Read the model definition and answer for the solid it produces. Units are mm, in the model's axes. Face numbers are marked on the shaded views. A direction names the side the tool comes from. Give positions to 0.01 mm unless a question says otherwise; leave off trailing zeros. Order: outer loops, then holes, each group sorted by start corner. A loop starts at its lowest first (then second) coordinate and runs counter-clockwise, first axis right, second up. Notation, with made-up numbers: (54.25, 88.25) - (86.25, 88.25) arc R25 ccw to (86.25, 103.25) - close; hole circle Ø4 at (-17.75, 21). An arc over 180 degrees is marked (long way). Write each question's results on one line, items separated by ' | '.
from build123d import *

# Parameters (mm, degrees)
BOSS_EXTRUDE3_DEPTH = 2
SKETCH1_6_W         = 100
SKETCH1_6_H         = 50
BOSS_EXTRUDE4_DEPTH = 5
SKETCH2_W           = 120
SKETCH2_H           = 65
SKETCH2_R           = 1.45
SKETCH2_R_2         = 1.6
BOSS_EXTRUDE5_DEPTH = 30
SKETCH2_2_W         = 120
SKETCH2_2_H         = 65
SKETCH2_2_R         = 1.45
SKETCH2_2_R_2       = 1.6
BOSS_EXTRUDE6_DEPTH = 3
CUT_EXTRUDE1_REACH  = 77.367
SKETCH7_W           = 43
SKETCH7_H           = 32
FILLET1_R           = 10


with BuildPart() as part:
    # Sketch1 → Boss-Extrude3 (new body)
    with BuildSketch(Plane(origin=(0, 0, 0), x_dir=(1, 0, 0), z_dir=(0, 1, 0))):
        Polygon((23, -14.25), (23, -17.5), (-23, -17.5), (-23, -14.25), (-38.5, -14.25), (-38.5, 14.25), (-23, 14.25), (-23, 17.5), (23, 17.5), (23, 14.25), (38.5, 14.25), (38.5, -14.25), align=None)
    extrude(amount=BOSS_EXTRUDE3_DEPTH)

    # Sketch1<6> → Boss-Extrude4 (add)
    with BuildSketch(Plane(origin=(0, 0, 0), x_dir=(1, 0, 0), z_dir=(0, 1, 0))):
        Rectangle(SKETCH1_6_W, SKETCH1_6_H)
        Polygon((23, -14.25), (23, -17.5), (-23, -17.5), (-23, -14.25), (-38.5, -14.25), (-38.5, 14.25), (-23, 14.25), (-23, 17.5), (23, 17.5), (23, 14.25), (38.5, 14.25), (38.5, -14.25), align=None, mode=Mode.SUBTRACT)
    extrude(amount=BOSS_EXTRUDE4_DEPTH)

    # Sketch2 → Boss-Extrude5 (add)
    with BuildSketch(Plane.XZ):
        Rectangle(SKETCH2_W, SKETCH2_H)
        with Locations(Location((-55, 28.75, 0), (0, 0, 270))):
            Circle(SKETCH2_R, mode=Mode.SUBTRACT)
        with Locations(Location((55, 28.75, 0), (0, 0, 90))):
            Circle(SKETCH2_R, mode=Mode.SUBTRACT)
        with Locations(Location((55, -28.75, 0), (0, 0, 270))):
            Circle(SKETCH2_R, mode=Mode.SUBTRACT)
        with Locations(Location((-55, -28.75, 0), (0, 0, 90))):
            Circle(SKETCH2_R, mode=Mode.SUBTRACT)
        with Locations(Location((50, 28.75, 0), (0, 0, 270))):
            Circle(SKETCH2_R_2, mode=Mode.SUBTRACT)
        with Locations(Location((50, -28.75, 0), (0, 0, 90))):
            Circle(SKETCH2_R_2, mode=Mode.SUBTRACT)
    extrude(amount=BOSS_EXTRUDE5_DEPTH)

    # Sketch2<2> → Boss-Extrude6 (add)
    with BuildSketch(Plane.XZ):
        Rectangle(SKETCH2_2_W, SKETCH2_2_H)
        with Locations(Location((-55, 28.75, 0), (0, 0, 270))):
            Circle(SKETCH2_2_R, mode=Mode.SUBTRACT)
        with Locations(Location((55, 28.75, 0), (0, 0, 90))):
            Circle(SKETCH2_2_R, mode=Mode.SUBTRACT)
        with Locations(Location((55, -28.75, 0), (0, 0, 270))):
            Circle(SKETCH2_2_R, mode=Mode.SUBTRACT)
        with Locations(Location((-55, -28.75, 0), (0, 0, 90))):
            Circle(SKETCH2_2_R, mode=Mode.SUBTRACT)
        with Locations(Location((50, 28.75, 0), (0, 0, 270))):
            Circle(SKETCH2_2_R_2, mode=Mode.SUBTRACT)
        with Locations(Location((50, -28.75, 0), (0, 0, 90))):
            Circle(SKETCH2_2_R_2, mode=Mode.SUBTRACT)
    extrude(amount=BOSS_EXTRUDE6_DEPTH)

    # Sketch7 → Cut-Extrude1 (cut, up to next)
    with BuildSketch(Plane(origin=(0, 2, 0), x_dir=(1, 0, 0), z_dir=(0, 1, 0)), mode=Mode.PRIVATE) as cut_extrude1_sk1:
        Rectangle(SKETCH7_W, SKETCH7_H)
    cut_extrude1_tool1 = extrude(cut_extrude1_sk1.sketch, amount=-CUT_EXTRUDE1_REACH, mode=Mode.PRIVATE) & part.part
    add(cut_extrude1_tool1.solids().sort_by_distance((0, 2, 0))[0], mode=Mode.SUBTRACT)

    # Fillet1
    # the kernel refuses this fillet: 10 mm, written as the material it takes off along each edge
    with BuildSketch(Plane(origin=(-21.5, 2, 16), x_dir=(0, -1, 0), z_dir=(0, 0, -1))) as fillet1_piece_1_section:
        with BuildLine():
            CenterArc((FILLET1_R, FILLET1_R), FILLET1_R, 180, 90)
            Line((0, FILLET1_R), (0, 0))
            Line((0, 0), (FILLET1_R, 0))
        make_face()
    fillet1_piece_1 = extrude(amount=32, mode=Mode.PRIVATE)
    fillet1_piece_1 = split(fillet1_piece_1, bisect_by=Plane(origin=(-23, -2.387167078, 15.125), z_dir=(1, 0, 0)), keep=Keep.TOP, mode=Mode.PRIVATE)
    add(fillet1_piece_1, mode=Mode.SUBTRACT)
    with BuildSketch(Plane(origin=(-21.5, 2, 41), x_dir=(0, -1, 0), z_dir=(0, 0, -1))) as fillet1_piece_2_section:
        with BuildLine():
            CenterArc((FILLET1_R, FILLET1_R), FILLET1_R, 180, 90)
            Line((0, FILLET1_R), (0, 0))
            Line((0, 0), (FILLET1_R, 0))
        make_face()
    fillet1_piece_2 = extrude(amount=82, mode=Mode.PRIVATE)
    fillet1_piece_2 = split(fillet1_piece_2, bisect_by=Plane(origin=(-23.780995079, -0.852225246, -14.25), z_dir=(0, 0, 1)), keep=Keep.TOP, mode=Mode.PRIVATE)
    fillet1_piece_2 = split(fillet1_piece_2, bisect_by=Plane(origin=(-23.780995079, -0.852225246, 14.25), z_dir=(0, 0, -1)), keep=Keep.TOP, mode=Mode.PRIVATE)
    add(fillet1_piece_2, mode=Mode.SUBTRACT)
    with BuildSketch(Plane(origin=(21.5, 2, -16), x_dir=(0, -1, 0), z_dir=(0, 0, 1))) as fillet1_piece_3_section:
        with BuildLine():
            CenterArc((FILLET1_R, FILLET1_R), FILLET1_R, 180, 90)
            Line((0, FILLET1_R), (0, 0))
            Line((0, 0), (FILLET1_R, 0))
        make_face()
    fillet1_piece_3 = extrude(amount=32, mode=Mode.PRIVATE)
    fillet1_piece_3 = split(fillet1_piece_3, bisect_by=Plane(origin=(23, -2.387167078, -15.125), z_dir=(-1, 0, 0)), keep=Keep.TOP, mode=Mode.PRIVATE)
    add(fillet1_piece_3, mode=Mode.SUBTRACT)
    with BuildSketch(Plane(origin=(21.5, 2, -41), x_dir=(0, -1, 0), z_dir=(0, 0, 1))) as fillet1_piece_4_section:
        with BuildLine():
            CenterArc((FILLET1_R, FILLET1_R), FILLET1_R, 180, 90)
            Line((0, FILLET1_R), (0, 0))
            Line((0, 0), (FILLET1_R, 0))
        make_face()
    fillet1_piece_4 = extrude(amount=82, mode=Mode.PRIVATE)
    fillet1_piece_4 = split(fillet1_piece_4, bisect_by=Plane(origin=(23.780995079, -0.852225246, 14.25), z_dir=(0, 0, -1)), keep=Keep.TOP, mode=Mode.PRIVATE)
    fillet1_piece_4 = split(fillet1_piece_4, bisect_by=Plane(origin=(23.780995079, -0.852225246, -14.25), z_dir=(0, 0, 1)), keep=Keep.TOP, mode=Mode.PRIVATE)
    add(fillet1_piece_4, mode=Mode.SUBTRACT)


solid = part.part
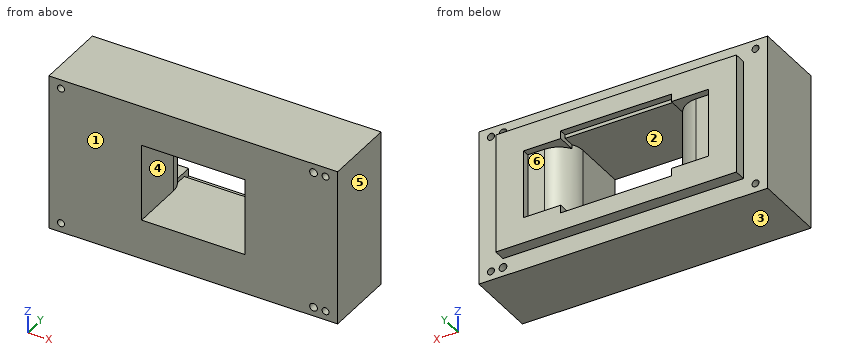
(1) The mould has two halves that part along Z. Classify the marked faces 1, 2 and 3: pulls with the +Z half, pulls with the -Z half, needs draft (parallel to the pull), parting line crosses it, or undercut.
Conclusion:
face 1: needs draft | face 2: undercut | face 3: pulls with the -Z half
(2) Section B-B (y = -15) is taken. Give the vertices of the cut face in (x, z), plus the area to 3 significant figures.
Conclusion:
outline: (-60, -32.5) - (60, -32.5) - (60, 32.5) - (-60, 32.5) - close; hole circle Ø2.9 at (-55, -28.75); hole circle Ø2.9 at (-55, 28.75); hole (-21.5, -16) - (21.5, -16) - (21.5, 16) - (-21.5, 16) - close; hole circle Ø3.2 at (50, -28.75); hole circle Ø3.2 at (50, 28.75); hole circle Ø2.9 at (55, -28.75); hole circle Ø2.9 at (55, 28.75) | area: 6,380 mm^2
(3) Section C-C (x = -55) is taken. Give the vertices of the cut face in (y, z).
Conclusion:
outline: (-30, -32.5) - (0, -32.5) - (0, -30.2) - (-30, -30.2) - close; (-30, -27.3) - (0, -27.3) - (0, 27.3) - (-30, 27.3) - close; (-30, 30.2) - (0, 30.2) - (0, 32.5) - (-30, 32.5) - close
(4) Each of these flat-tipped pins is pushed along its axis until it touches: pin 1 (1.5 mm diameter, centred on y = 3.5, z = 4.5, fed in from -X); pin 2 (4 mm diameter, centred on x = 50, z = -28.75, fed in from +Y); pin 3 (1.5 mm diameter, centred on y = 3, z = -3.5, fed in from +X); pin 4 (5 mm diameter, centred on x = -18, z = 4, fed in from -Y) (1 decimal). Where does it stop, or does it pass through?
Conclusion:
pin 1: x = -50 | pin 2: y = 0 | pin 3: x = 50 | pin 4: through
(5) For the marked faces 4, 5 and 6, determine the directions among +Z, -Z, +X, -X, +Y, -Y from which every point of the face is accessible in a straight line to the end or side of a thin tool.
Conclusion:
face 4: +Y, -Y | face 5: +Z, -Z, +X, +Y, -Y | face 6: +Y
(6) Section D-D (z = -28.75) is taken. Give the vertices of the cut face in (x, y), plus the area to 3 significant figures.
Conclusion:
outline: (-60, -30) - (-56.45, -30) - (-56.45, 0) - (-60, 0) - close; (-53.55, -30) - (48.4, -30) - (48.4, 0) - (-53.55, 0) - close; (51.6, -30) - (53.55, -30) - (53.55, 0) - (51.6, 0) - close; (56.45, -30) - (60, -30) - (60, 0) - (56.45, 0) - close | area: 3,330 mm^2
(7) Section A-A (z = 1) is taken. Give the vertices of the cut face in (x, y).
Conclusion:
outline: (-60, -30) - (-21.5, -30) - (-21.5, -8) arc R10 ccw to (-31.5, 2) - (-38.5, 2) - (-38.5, 5) - (-50, 5) - (-50, 0) - (-60, 0) - close; (21.5, -30) - (60, -30) - (60, 0) - (50, 0) - (50, 5) - (38.5, 5) - (38.5, 2) - (31.5, 2) arc R10 ccw to (21.5, -8) - close
(8) Consider probe 1 along X at (y, z) = (-18, -28.75); probe 2 along X at (y, z) = (-21, -4); probe 3 along Z at (x, y) = (-9, 4). Determine where each line is inside the solid, lowest interval first. Write a range as [from, to].
Conclusion:
probe 1: [-60, -56.45], [-53.55, 48.4], [51.6, 53.55], [56.45, 60] | probe 2: [-60, -21.5], [21.5, 60] | probe 3: [-25, -17.5], [17.5, 25]
